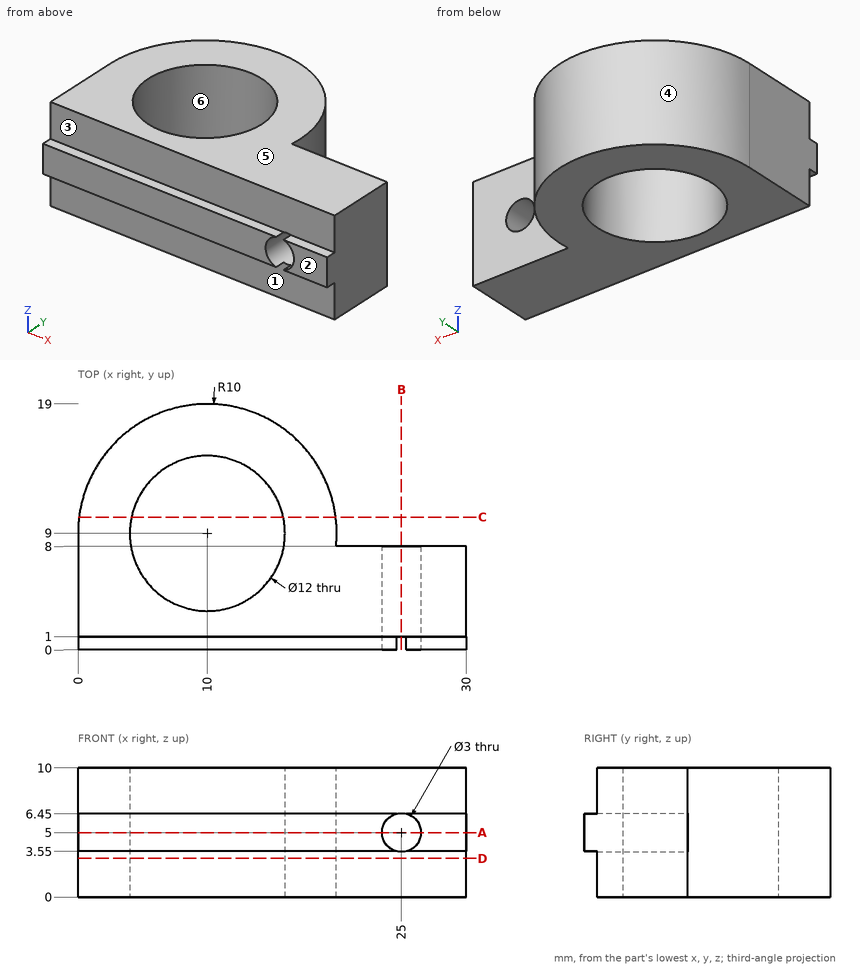
The drawing under review shows one solid part. Ordinate dimensions are in mm from its lowest x, y, z. A direction names the side the tool comes from. Coordinates: 2 decimals unless noted, no trailing zeros. Order: outer loops, then holes, each group sorted by start corner. A loop starts at its lowest first (then second) coordinate and runs counter-clockwise, first axis right, second up. Notation, with made-up numbers: (11.25, -4.75) -> (18.25, -4.75) arc R5 cw to (18.25, 2.25) -> close; hole circle Ø2 at (7.25, 3). An arc over 180 degrees is marked (long way). Use CSV: the item, a comma, the result in double quotes. Start each with the question number.
Item 1: Wall thickness on probe 1 along X at (y, z) = (2.5, 5); probe 2 along Y at (x, z) = (10, 5.5); probe 3 along X at (y, z) = (5, 5): over which ranges is each line inside the solid? List them lowest first.
Item 2: We need section C-C, the plane y = 10.25. Give the boundary of the cut face in (x, z).
Item 3: Insertion check: pin 1 (2 mm diameter, centred on x = 22.5, z = 6.5, fed in from +Y); pin 2 (2 mm diameter, centred on y = 16, z = 4, fed in from -X); pin 3 (0.5 mm diameter, centred on x = 28.5, y = 0.5, fed in from +Z); pin 4 (2.5 mm diameter, centred on x = 25, z = 5, fed in from +Y). Each pin has a flat end and moves straight along its axis. Give the tip position at first contact, or say it passes through.
Item 4: We need section D-D, the plane z = 3. Give the boundary of the cut face in (x, y), then the cut area to 3 significant figures.
Item 5: We need section A-A, the plane z = 5. Give the boundary of the cut face in (x, y), then the cut area to 3 significant figures.
Item 6: We need section B-B, the plane x = 25. Give the boundary of the cut face in (y, z).
Item 7: For the marked faces 1, 2 and 3, list the 3-axis set-ups (+Z, -Z, +X, -X, +Y, -Y) from which the entire face can be reached by the end or side of a thin tool; tool diameter is ignored.
Item 8: Draft analysis for pull direction X (two halves, no side actions). For the marked faces 4, 5 and 6, state which applies: pulls with the +X half, pulls with the -X half, needs draft (parallel to the pull), parting line crosses it, or undercut.
Derived:
1,probe 1,"x = 0 to 23.5, 26.5 to 30"
1,probe 2,"y = 0 to 3, 15 to 19"
1,probe 3,"x = 0 to 5.53, 14.47 to 23.5, 26.5 to 30"
2,outline,"(0.08, 0) -> (4.13, 0) -> (4.13, 10) -> (0.08, 10) -> close; (15.87, 0) -> (19.92, 0) -> (19.92, 10) -> (15.87, 10) -> close"
3,pin 1,"stops at y = 8"
3,pin 2,"stops at x = 2"
3,pin 3,"stops at z = 6.45"
3,pin 4,"passes through"
4,outline,"(0, 1) -> (30, 1) -> (30, 8) -> (19.95, 8) arc R10 ccw (long way) to (0, 9) -> close; hole circle Ø12 at (10, 9)"
4,area,"274 mm^2"
5,outline,"(0, 0) -> (23.5, 0) -> (23.5, 8) -> (19.95, 8) arc R10 ccw (long way) to (0, 9) -> close; (26.5, 0) -> (30, 0) -> (30, 8) -> (26.5, 8) -> close; hole circle Ø12 at (10, 9)"
5,area,"280 mm^2"
6,outline,"(1, 0) -> (8, 0) -> (8, 3.5) -> (1, 3.5) -> close; (1, 6.5) -> (8, 6.5) -> (8, 10) -> (1, 10) -> close"
7,face 1,"-Z, +X, -X, -Y"
7,face 2,"+Z, -Z, +X, -X, -Y"
7,face 3,"+Z, +X, -X, -Y"
8,face 4,"parting line crosses it"
8,face 5,"needs draft"
8,face 6,"undercut"
